Part model, mm, in its own coordinate system. Face numbers are marked on the shaded views. A direction names the side the tool comes from. Give positions to 0.01 mm unless a question says otherwise; leave off trailing zeros. Loops run counter-clockwise (first coordinate to the right, second up) from the corner with the lowest first, then second, coordinate; pieces in that order, holes last. Notation, with made-up numbers: (-21.5, -38) -> (10.5, -38) arc R27 ccw to (10.5, -12) -> close; hole circle Ø10 at (71.25, 79.25). An arc over 180 degrees is marked (long way). One line per question, with ' | ' between items.
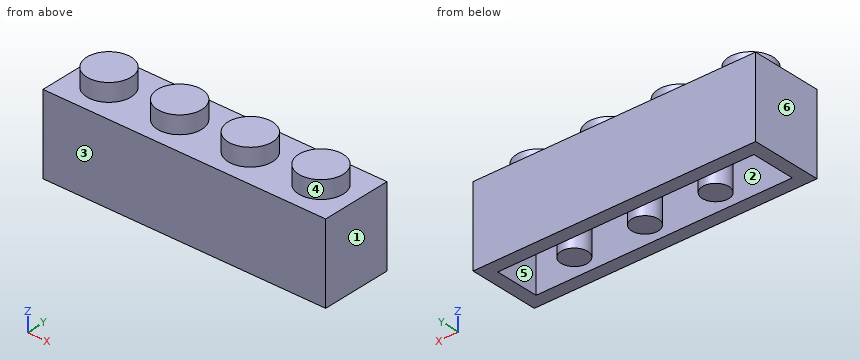
```python
from build123d import *

# Parameters (mm, degrees)
F0_W     = 32
F0_H     = 9
F1_DEPTH = 8
F2_R     = 2.5
F3_DEPTH = 2
F4_W     = 29
F4_H     = 5
F4_R     = 1.5
F5_DEPTH = 8
F6_R     = 1.25
F7_DEPTH = 10


with BuildPart() as f1:
    # F0 (on Front) → F1 (new body)
    with BuildSketch(Plane.XZ):
        Rectangle(F0_W, F0_H)
    extrude(amount=-F1_DEPTH)

    # F2 (on face) → F3 (join)
    with BuildSketch(Plane.XY.offset(4.5)):
        with Locations((-12, 4)):
            Circle(F2_R)
        with Locations((-4, 4)):
            Circle(F2_R)
        with Locations((4, 4)):
            Circle(F2_R)
        with Locations((12, 4)):
            Circle(F2_R)
    extrude(amount=F3_DEPTH)

    # F4 (on face) → F5 (cut)
    with BuildSketch(Plane(origin=(0, 0, -4.5), x_dir=(1, 0, 0), z_dir=(0, 0, -1))):
        with Locations((0, -4)):
            Rectangle(F4_W, F4_H)
        with Locations((-8, -4)):
            Circle(F4_R, mode=Mode.SUBTRACT)
        with Locations((0, -4)):
            Circle(F4_R, mode=Mode.SUBTRACT)
        with Locations((8, -4)):
            Circle(F4_R, mode=Mode.SUBTRACT)
    extrude(amount=-F5_DEPTH, mode=Mode.SUBTRACT)

    # F6 (on face) → F7 (cut)
    with BuildSketch(Plane(origin=(0, 0, -4.5), x_dir=(1, 0, 0), z_dir=(0, 0, -1))):
        with Locations((-12, -4)):
            Circle(F6_R)
        with Locations((-4, -4)):
            Circle(F6_R)
        with Locations((4, -4)):
            Circle(F6_R)
        with Locations((12, -4)):
            Circle(F6_R)
    extrude(amount=-F7_DEPTH, mode=Mode.SUBTRACT)


solid = f1.part
```
1) Drill centre lines: line 1 (Y direction, x = -4, z = 4.15); line 2 (Y direction, x = -8.5, z = -1); line 3 (X direction, y = 3, z = 4). Where is each one in solid material? Low to high.
Found:
line 1: 0 to 2.75, 5.25 to 8 | line 2: 0 to 1.5, 2.59 to 5.41, 6.5 to 8 | line 3: -16 to -12.75, -11.25 to -4.75, -3.25 to 3.25, 4.75 to 11.25, 12.75 to 16
2) Pull direction Y, two halves, no side cores. Call the marked faces 1, 2 and 3: pulls with the +Y half, pulls with the -Y half, needs draft (parallel to the pull), parting line crosses it, or undercut.
Found:
face 1: needs draft | face 2: undercut | face 3: pulls with the -Y half
3) Saw through at D-D (y = 6). Give the cut face in (x, z).
Found:
outline: (-16, -4.5) -> (-14.5, -4.5) -> (-14.5, 3.5) -> (14.5, 3.5) -> (14.5, -4.5) -> (16, -4.5) -> (16, 4.5) -> (13.5, 4.5) -> (13.5, 6.5) -> (10.5, 6.5) -> (10.5, 4.5) -> (5.5, 4.5) -> (5.5, 6.5) -> (2.5, 6.5) -> (2.5, 4.5) -> (-2.5, 4.5) -> (-2.5, 6.5) -> (-5.5, 6.5) -> (-5.5, 4.5) -> (-10.5, 4.5) -> (-10.5, 6.5) -> (-13.5, 6.5) -> (-13.5, 4.5) -> (-16, 4.5) -> close
4) Saw through at C-C (x = 4). Give the cut face in (y, z).
Found:
outline: (0, -4.5) -> (1.5, -4.5) -> (1.5, 3.5) -> (2.75, 3.5) -> (2.75, 5.5) -> (5.25, 5.5) -> (5.25, 3.5) -> (6.5, 3.5) -> (6.5, -4.5) -> (8, -4.5) -> (8, 4.5) -> (6.5, 4.5) -> (6.5, 6.5) -> (1.5, 6.5) -> (1.5, 4.5) -> (0, 4.5) -> close
5) Pin check, flat tips, straight feed: P1, Ø2, axis at x = 12, y = 4, coming from the -Z side; P2, Ø3, axis at x = 4.5, y = 3.5, coming from the -Z side. Stop position of each tip, or through.
Found:
P1: z = 5.5 | P2: z = 3.5
6) Tool access for the marked faces 4, 5 and 6: list every direction of +Z, -Z, +X, -X, +Y, -Y with a clear straight run to the whole face (end or side of a thin tool).
Found:
face 4: +Z | face 5: -Z | face 6: +Z, -Z, -X, +Y, -Y
7) Saw through at B-B (z = 4). Give the cut face in (x, y).
Found:
outline: (-16, 0) -> (16, 0) -> (16, 8) -> (-16, 8) -> close; hole circle Ø2.5 at (-12, 4); hole circle Ø2.5 at (-4, 4); hole circle Ø2.5 at (4, 4); hole circle Ø2.5 at (12, 4)
8) Saw through at A-A (z = -0.5). Give the cut face in (x, y), and give its area (3 significant figures).
Found:
outline: (-16, 0) -> (16, 0) -> (16, 8) -> (-16, 8) -> close; circle Ø3 at (-8, 4); circle Ø3 at (0, 4); circle Ø3 at (8, 4); hole (-14.5, 1.5) -> (14.5, 1.5) -> (14.5, 6.5) -> (-14.5, 6.5) -> close | area: 132 mm2
